Verification items for this drawing (mm, ordinates from the low corner). Round coordinates to 2 decimals unless told otherwise and drop trailing zeros. Write each loop counter-clockwise with the first axis right and the second up, starting at its lowest first coordinate (ties: lowest second). Pieces come first, ordered by that corner, then holes. Notation, with made-up numbers: M 65.5,-35 L 77.5,-35 A19 ccw 77.5,-27 Z; hole C -16,-30 d9. An arc over 180 degrees is marked long. One line per question, with ' | ' between items. Start each with the question number.
Q1. Cross-section at B-B (x = 90). Record the boundary of the cut face in (y, z) (1 decimal).
Q2. Thickness scan on line 1 along X through (y, z) = (0.85, 68); line 2 along X through (y, z) = (9, 136.5); line 3 along Z through (x, y) = (125, 0.8). Record the ranges inside material, lowest first. Write a range as from..to.
Q3. Release check for a two-part mould opening along X. For the marked faces 1 and 2 record: released by +X, released by -X, zero draft, split by the parting line, or undercut.
Q4. Cross-section at A-A (z = 68). Record the boundary of the cut face in (x, y), then the cut area to 3 significant figures.
Q5. Gauge pin test, flat end, axial feed: pin 1 (3 mm diameter, centred on x = 20, y = 4, fed in from -Z). Record the tip position at first contact, or that the pin passes through.
Q6. Cross-section at C-C (z = 28.5). Record the boundary of the cut face in (x, y).
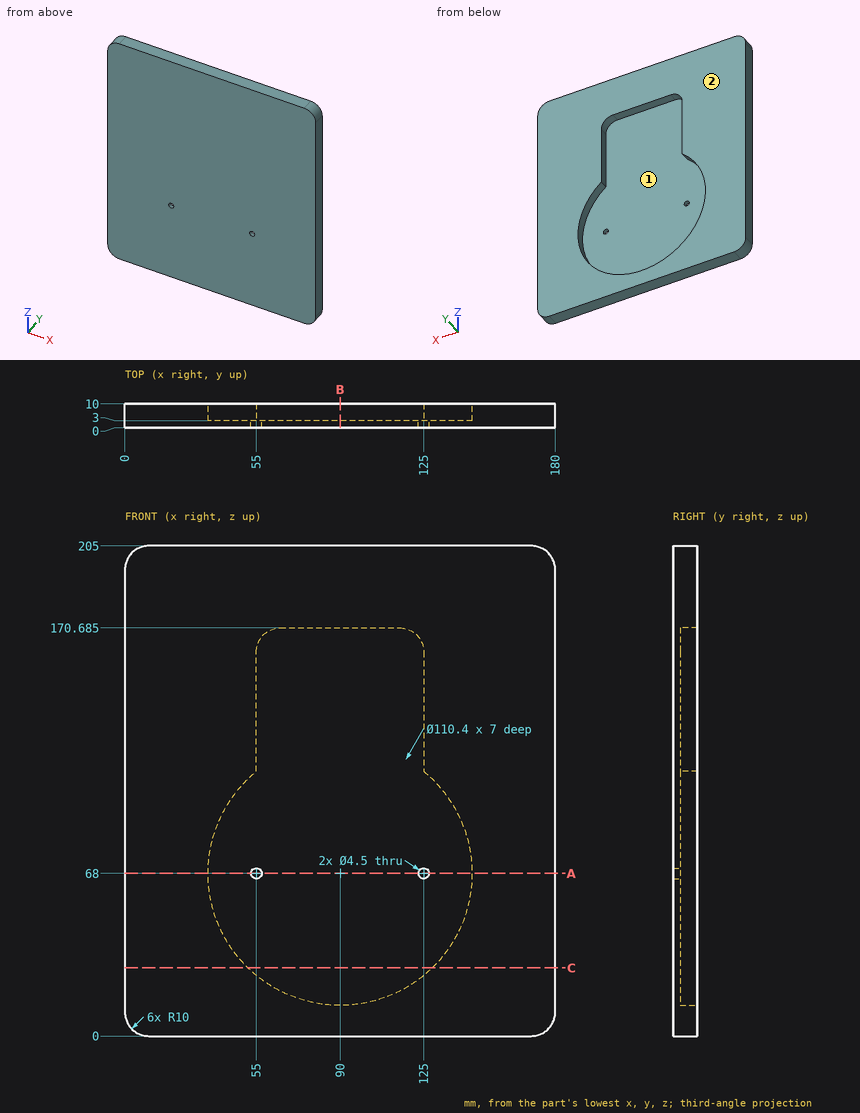
Determined:
1) outline: M 0,0 L 10,0 L 10,12.8 L 3,12.8 L 3,170.7 L 10,170.7 L 10,205 L 0,205 Z
2) line 1: x = 0..52.75, 57.25..122.75, 127.25..180 | line 2: x = 0..55, 125..180 | line 3: z = 0..65.75, 70.25..205
3) face 1: undercut | face 2: zero draft
4) outline: M 0,0 L 52.75,0 L 52.75,3 L 34.8,3 L 34.8,10 L 0,10 Z; M 57.25,0 L 122.75,0 L 122.75,3 L 57.25,3 Z; M 127.25,0 L 180,0 L 180,10 L 145.2,10 L 145.2,3 L 127.25,3 Z | area: 1,000 mm²
5) pin 1: stops at z = 0
6) outline: M 0,0 L 180,0 L 180,10 L 128.56,10 L 128.56,3 L 51.44,3 L 51.44,10 L 0,10 Z
